Read the model definition and answer for the solid it produces. Units are mm, in the model's axes. Face numbers are marked on the shaded views. Give positions to 0.01 mm unless a question says otherwise; leave off trailing zeros. Order: outer loops, then holes, each group sorted by start corner. A loop starts at its lowest first (then second) coordinate and runs counter-clockwise, first axis right, second up.
Item 1: Find the intervals of material crossed by line 1 along Y through (x, z) = (0, 2); line 2 along Y through (x, z) = (37, 3.25); line 3 along Y through (x, z) = (-54.5, 8.5), in increasing order.
Item 2: A cutting plane is placed at D-D (y = -62). Write down the section's boundary in (x, z), plus the area to 3 significant figures.
Item 3: Given pin 1 Ø2 at (x, z) = (-2, 2.5) entering from -Y; pin 2 Ø1 at (y, z) = (4.5, 6.5) entering from -X; pin 3 Ø3 at (y, z) = (-79, 3) entering from -X, each flat-ended and moving along its own axis, determine where each tip first touches the part or whether it passes through.
Item 4: A cutting plane is placed at B-B (x = 54). Write down the section's boundary in (y, z), plus the area to 3 significant figures.
Item 5: A cutting plane is placed at A-A (z = 2). Write down the section's boundary in (x, y).
Item 6: The mould has two halves that part along Y. Classify the marked faces 1, 2, 3 and 4: +Y half, -Y half, draft (parallel to the pull), parting line (faces both ways), or undercut.
Item 7: A cutting plane is placed at C-C (y = 8). Write down the section's boundary in (x, z), plus the area to 3 significant figures.
Autodesk Inventor part; units mm, degrees
ref_plane "YZ Plane" through (0, 0, 0) normal (1, 0, 0) x (0, 1, 0)
ref_plane "XZ Plane" through (0, 0, 0) normal (0, 1, 0) x (-1, 0, 0)
ref_plane "XY Plane" through (0, 0, 0) normal (0, 0, 1) x (1, 0, 0)
sketch "Sketch1" plane through (0, 0, 0) normal (0, 0, 1) x (1, 0, 0)
  circle A0 centre (0, 0) radius 28 construction
  line L0 (75, -135) -> (-75, -135) construction
  line L1 (-75, -135) -> (-75, 65) construction
  line L2 (-75, 65) -> (75, 65) construction
  line L3 (75, 65) -> (75, -135) construction
  line L4 (75, -135) -> (-75, 65) construction
  line L5 (-75, -135) -> (75, 65) construction
  circle A1 centre (0, 0) radius 20
  circle A2 centre (-38.9711, -22.5) radius 20
  circle A3 centre (-38.9711, -67.5) radius 20
  circle A4 centre (0, -90) radius 20
  circle A5 centre (38.9711, -67.5) radius 20
  circle A6 centre (38.9711, -22.5) radius 20
  circle A7 centre (0, -45) radius 67.5
  circle A8 centre (0, -45) radius 1.5
  circle A9 centre (0, -45) radius 4.05
  point P0 (0, -35)
  dimension "d0" = 56
  dimension "d1" = 150
  dimension "d2" = 200
  dimension "d3" = 135
  dimension "d4" = 40
  dimension "d7" = 360
  dimension "d9" = 45
  dimension "d10" = 135
  dimension "d11" = 3
  dimension "d12" = 8.1
extrude "Extrusion1" add sketch "Sketch1" along normal blind 10 contours A7
extrude "Extrusion2" add sketch "Sketch1" along normal blind 7 contours A9
properties part number "FilterWheel-M40-6pos"
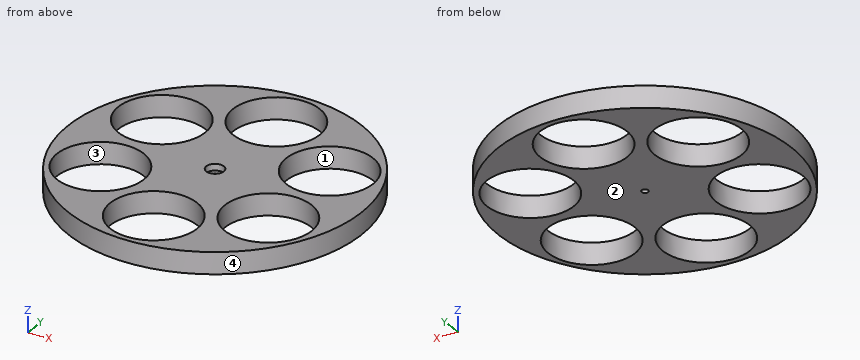
Response values:
1. line 1: y = -112.5 to -110, -70 to -46.5, -43.5 to -20, 20 to 22.5
1. line 2: y = -101.46 to -87.4, -47.6 to -42.4, -2.6 to 11.46
1. line 3: y = -84.82 to -80.1, -54.9 to -35.1, -9.9 to -5.18
2. outline: (-65.32, 0) - (-58.2, 0) - (-58.2, 10) - (-65.32, 10) - close; (-19.74, 0) - (19.74, 0) - (19.74, 10) - (-19.74, 10) - close; (58.2, 0) - (65.32, 0) - (65.32, 10) - (58.2, 10) - close
2. area: 537 mm2
3. pin 1: stops at y = -112.49
3. pin 2: stops at x = -46.42
3. pin 3: stops at x = -59.16
4. outline: (-85.5, 0) - (-80.7, 0) - (-80.7, 10) - (-85.5, 10) - close; (-54.3, 0) - (-35.7, 0) - (-35.7, 10) - (-54.3, 10) - close; (-9.3, 0) - (-4.5, 0) - (-4.5, 10) - (-9.3, 10) - close
4. area: 282 mm2
5. outline: circle Ø135 at (0, -45); hole circle Ø40 at (-38.97, -67.5); hole circle Ø40 at (-38.97, -22.5); hole circle Ø40 at (0, -90); hole circle Ø40 at (0, 0); hole circle Ø3 at (0, -45); hole circle Ø40 at (38.97, -67.5); hole circle Ø40 at (38.97, -22.5)
6. face 1: undercut
6. face 2: draft
6. face 3: undercut
6. face 4: parting line
7. outline: (-41.8, 0) - (-18.33, 0) - (-18.33, 10) - (-41.8, 10) - close; (18.33, 0) - (41.8, 0) - (41.8, 10) - (18.33, 10) - close
7. area: 469 mm2
